from build123d import *

# Parameters (mm, degrees)
F0_W     = 34.925
F0_H     = 50.8
F1_DEPTH = 3.175
F3_D     = 2.2606
F3_DEPTH = 27.305
F3_TIP   = 0.6791527577


with BuildPart() as f1:
    # F0 (on Right) → F1 (new body, symmetric)
    with BuildSketch(Plane.YZ):
        Rectangle(F0_W, F0_H)
    extrude(amount=F1_DEPTH, both=True)

    # F3
    with Locations(Plane(origin=(0, 0, -25.4), x_dir=(1, 0, 0), z_dir=(0, 0, -1))):
        with Locations((0, 12.7), (0, -12.7)):
            Hole(F3_D / 2, depth=F3_DEPTH)
            with Locations((0, 0, -(F3_DEPTH + F3_TIP / 2))):  # 118° drill point
                Cone(0, F3_D / 2, F3_TIP, mode=Mode.SUBTRACT)


solid = f1.part
Model file for the job. Use its own axes, mm. A direction names the side the tool comes from. Coordinates: 2 decimals unless noted, no trailing zeros. Order: outer loops, then holes, each group sorted by start corner. A loop starts at its lowest first (then second) coordinate and runs counter-clockwise, first axis right, second up. Notation, with made-up numbers: (38, -12.75) -> (83, -12.75) arc R8 ccw to (83, -4.75) -> close; hole circle Ø5 at (30, -1). An arc over 180 degrees is marked (long way). Return JSON: item names as keys, results as strings. Group by question number.
Item 1: Saw through at A-A on z = -16. Write the cut outline in (x, y) (1 decimal).
Item 2: Tool access for faces 4 (the cylindrical face through (0.15, -13.82, -11.56)), 5 (the flat face through (0, -17.462, 0)): list every direction of +Z, -Z, +X, -X, +Y, -Y with a clear straight run to the whole face (end or side of a thin tool).
Item 3: Wall check: line 1 along Y through (x, z) = (0, -18.75); line 2 along X through (y, z) = (12.7, -19.5) (3 decimals); line 3 along Y through (x, z) = (0.75, -16). Give the ranges that are in metal, low to high. Write a range as [from, to].
Item 4: Pull direction X, two halves, no side cores. Call faces 1 (the conical face through (0.106, -12.866, 2.466)), 2 (the flat face through (3.175, 0, 0)), 3 (the flat face through (-3.175, 0, 0)): pulls with the +X half, pulls with the -X half, needs draft (parallel to the pull), parting line crosses it, or undercut.
Values found:
{
 "1": {"outline": "(-3.2, -17.5) -> (3.2, -17.5) -> (3.2, 17.5) -> (-3.2, 17.5) -> close; hole circle Ø2.3 at (0, -12.7); hole circle Ø2.3 at (0, 12.7)"},
 "2": {"face 4": "-Z", "face 5": "+Z, -Z, +X, -X, -Y"},
 "3": {"line 1": "y = [-17.46, -13.83], [-11.57, 11.57], [13.83, 17.46]", "line 2": "x = [-3.175, -1.13], [1.13, 3.175]", "line 3": "y = [-17.46, -13.55], [-11.85, 11.85], [13.55, 17.46]"},
 "4": {"face 1": "undercut", "face 2": "pulls with the +X half", "face 3": "pulls with the -X half"}
}
